```python
from build123d import *

# Parameters (mm, degrees)
BOSS_EXTRUDE4_DEPTH = 60
BOSS_EXTRUDE5_DEPTH = 51


with BuildPart() as part:
    # Sketch8 → Boss-Extrude4 (new body)
    with BuildSketch(Plane(origin=(0, 58, 0), x_dir=(1, 0, 0), z_dir=(0, 1, 0))):
        with BuildLine():
            Line((-15, -12), (15, -12))
            ThreePointArc((15, -12), (16.414213562, -11.414213562), (17, -10))
            Line((17, -10), (17, 10))
            ThreePointArc((17, 10), (16.414213562, 11.414213562), (15, 12))
            Line((15, 12), (-15, 12))
            ThreePointArc((-15, 12), (-16.414213562, 11.414213562), (-17, 10))
            Line((-17, 10), (-17, -10))
            ThreePointArc((-17, -10), (-16.414213562, -11.414213562), (-15, -12))
        make_face()
        with BuildLine():
            Line((-13, -10), (13, -10))
            ThreePointArc((13, -10), (14.414213562, -9.414213562), (15, -8))
            Line((15, -8), (15, 8))
            ThreePointArc((15, 8), (14.414213562, 9.414213562), (13, 10))
            Line((13, 10), (-13, 10))
            ThreePointArc((-13, 10), (-14.414213562, 9.414213562), (-15, 8))
            Line((-15, 8), (-15, -8))
            ThreePointArc((-15, -8), (-14.414213562, -9.414213562), (-13, -10))
        make_face(mode=Mode.SUBTRACT)
    extrude(amount=BOSS_EXTRUDE4_DEPTH)

    # Sketch11 → Boss-Extrude5 (add)
    with BuildSketch(Plane(origin=(0, 58, 0), x_dir=(1, 0, 0), z_dir=(0, 1, 0))):
        with BuildLine():
            Line((13, 10), (15, 10))
            Line((15, 10), (15, 6.937911183))
            Line((15, 6.937911183), (13.5, 6.937911183))
            ThreePointArc((13.5, 6.937911183), (13.146446609, 7.084357793), (13, 7.437911183))
            Line((13, 7.437911183), (13, 10))
        make_face()
        with BuildLine():
            Line((-13, 10), (-15, 10))
            Line((-15, 10), (-15, 8))
            Line((-15, 8), (-14, 8))
            ThreePointArc((-14, 8), (-13.292893219, 8.292893219), (-13, 9))
            Line((-13, 9), (-13, 10))
        make_face()
    extrude(amount=BOSS_EXTRUDE5_DEPTH)


solid = part.part
```
Geometry check sheet. Reference: the model listing, model coordinates, mm. A direction names the side the tool comes from. Give positions to 0.01 mm unless a question says otherwise; leave off trailing zeros. Loops run counter-clockwise (first coordinate to the right, second up) from the corner with the lowest first, then second, coordinate; pieces in that order, holes last. Notation, with made-up numbers: M 16,-28 L 65,-28 A27 cw 65,10 Z; hole C 75,56.25 d11. An arc over 180 degrees is marked long. Write item = value, one per line.
(1) Gauge pin test, flat ends, axial feed: pin 1 Ø8 at (x, z) = (-7.5, 0.5) entering from -Y; pin 2 Ø2 at (x, z) = (-14, -9) entering from +Y; pin 3 Ø0.6 at (x, z) = (13.5, -8.5) entering from +Y. Record the tip position at first contact, or that the pin passes through.
Answer below:
pin_1 = through
pin_2 = 118
pin_3 = 109
(2) Material ranges on line 1 (X direction, y = 63, z = -0.25); line 2 (Z direction, x = 7, y = 86); line 3 (Z direction, x = -14.5, y = 106.5), recorded low to high. Write a range as [from, to].
Answer below:
line_1 = [-17, -15], [15, 17]
line_2 = [-12, -10], [10, 12]
line_3 = [-12, -8], [9.32, 12]
(3) Release check for a two-part mould opening along Z. For faces 1 (the face through (-14.4, 113.44, -9.43)), 2 (the face through (0, 58, 11)), 3 (the face through (0, 88, -12)), 4 (the face through (0, 88, 12)) record: released by +Z, released by -Z, zero draft, split by the parting line, or undercut.
Answer below:
face_1 = undercut
face_2 = zero draft
face_3 = released by -Z
face_4 = released by +Z
(4) Sectioned sample at C-C, the plane z = 6.25. Record the cut outline in (x, y).
Answer below:
outline = M -17,58 L -15,58 L -15,118 L -17,118 Z; M 15,58 L 17,58 L 17,118 L 15,118 Z
(5) Sectioned sample at B-B, the plane x = -11. Record the cut outline in (y, z), plus the area to 3 significant figures.
Answer below:
outline = M 58,-12 L 118,-12 L 118,-10 L 58,-10 Z; M 58,10 L 118,10 L 118,12 L 58,12 Z
area = 240 mm2
(6) Tool access check on faces 5 (the face through (14, 109, -8)), 6 (the face through (14, 83, -6.938)), 7 (the face through (-16.43, 87.58, 11.4)). Record the directions out of +Z, -Z, +X, -X, +Y, -Y that give a thin tool (end or side, any length) a straight path to the whole face; none if there is none.
Answer below:
face_5 = +Y
face_6 = +Y, -Y
face_7 = +Z, -X, +Y, -Y
(7) Sectioned sample at D-D, the plane y = 80. Record the cut outline in (x, z), plus the area to 3 significant figures.
Answer below:
outline = M -17,-10 A2 ccw -15,-12 L 15,-12 A2 ccw 17,-10 L 17,10 A2 ccw 15,12 L -15,12 A2 ccw -17,10 Z; hole M -15,-8 L -14,-8 A1 cw -13,-9 L -13,-10 L 13,-10 L 13,-7.44 A0.5 cw 13.5,-6.94 L 15,-6.94 L 15,8 A2 ccw 13,10 L -13,10 A2 ccw -15,8 Z
area = 224 mm2
(8) Sectioned sample at A-A, the plane y = 113.5. Record the cut outline in (x, z).
Answer below:
outline = M -17,-10 A2 ccw -15,-12 L 15,-12 A2 ccw 17,-10 L 17,10 A2 ccw 15,12 L -15,12 A2 ccw -17,10 Z; hole M -15,-8 A2 ccw -13,-10 L 13,-10 A2 ccw 15,-8 L 15,8 A2 ccw 13,10 L -13,10 A2 ccw -15,8 Z
